from build123d import *

# Parameters (mm, degrees)
SKETCH_2_R        = 3.5
EXTRUDE_1_DEPTH   = 16
EXTRUDE_1_2_DEPTH = 16
EXTRUDE_1_3_DEPTH = 16
EXTRUDE_1_4_DEPTH = 16
SKETCH_3_W        = 288.1
SKETCH_3_H        = 15.5
EXTRUDE_2_DEPTH   = 15.5


with BuildPart() as part:
    # Sketch 2 → Extrude 1 (new body)
    with BuildSketch(Plane.XY):
        with Locations((-164, 0)):
            Circle(SKETCH_2_R)
    extrude(amount=EXTRUDE_1_DEPTH)



with BuildPart() as body_2:
    # Sketch 2 → Extrude 1 2 (new body)
    with BuildSketch(Plane.XY):
        with Locations((24.1, 0)):
            Circle(SKETCH_2_R)
    extrude(amount=EXTRUDE_1_2_DEPTH)


with BuildPart() as body_3:
    # Sketch 2 → Extrude 1 3 (new body)
    with BuildSketch(Plane.XY):
        with Locations((-204, 0)):
            Circle(SKETCH_2_R)
    extrude(amount=EXTRUDE_1_3_DEPTH)


with BuildPart() as body_4:
    # Sketch 2 → Extrude 1 4 (new body)
    with BuildSketch(Plane.XY):
        with Locations((64.1, 0)):
            Circle(SKETCH_2_R)
    extrude(amount=EXTRUDE_1_4_DEPTH)


with BuildPart() as part_1:
    add(part.part)

    add(body_2.part)  # Extrude 2 merges body 2

    add(body_3.part)  # Extrude 2 merges body 3

    add(body_4.part)  # Extrude 2 merges body 4
    # Sketch 3 → Extrude 2 (add)
    with BuildSketch(Plane(origin=(0, 0, 0), x_dir=(-1, 0, 0), z_dir=(0, 0, -1))):
        with Locations((69.95, 0)):
            Rectangle(SKETCH_3_W, SKETCH_3_H)
    extrude(amount=EXTRUDE_2_DEPTH)


solid = part_1.part
Work out the finished part from the listing and answer in its coordinate system (mm). A direction names the side the tool comes from. Give positions to 0.01 mm unless a question says otherwise; leave off trailing zeros. Order: outer loops, then holes, each group sorted by start corner. A loop starts at its lowest first (then second) coordinate and runs counter-clockwise, first axis right, second up. Notation, with made-up numbers: (39, -30) -> (93, -30) arc R23 ccw to (93, -5) -> close; hole circle Ø2 at (-9, 19). An arc over 180 degrees is marked (long way). Answer as a JSON object with one key per item and string values. Group by question number.
1. Section B-B on y = 0 is taken. Determine the outline of the cut face in (x, z), plus the area to 3 significant figures.
2. The mould has two halves that part along X. Classify faces 3 (the flat face through (24, 0, 16)), 4 (the cylindrical face through (67.333, -1.341, 7.888)), 5 (the flat face through (-214, 0, -8)), 6 (the flat face through (74.1, 0, -8)): released by +X, released by -X, zero draft, split by the parting line, or undercut.
3. Consider line 1 along X through (y, z) = (0.25, 1.5); line 2 along X through (y, z) = (3, 2.5); line 3 along Z through (x, y) = (-158, 0.5). Determine where each line is inside the solid, lowest interval first. Write a range as [from, to].
4. Section D-D on x = -125 is taken. Determine the outline of the cut face in (y, z), plus the area to 3 significant figures.
5. Section A-A on z = 11 is taken. Determine the outline of the cut face in (x, y), plus the area to 3 significant figures.
6. Section C-C on x = 64.1 is taken. Determine the outline of the cut face in (y, z), plus the area to 3 significant figures.
7. A flat-ended cylindrical pin translates along its axis: pin 1 Ø12 at (x, z) = (-146, 5) entering from +Y. Find the tip coordinate at first contact, or state that the pin passes through.
8. A tool of negligible diameter and unlimited length cuts with its end or side. For faces 1 (the cylindrical face through (-160.66, 1.05, 7.89)), 2 (the flat face through (64, 0, 16)), from which of +Z, -Z, +X, -X, +Y, -Y can it reach the whole face along a straight path? Write none if from no direction.
Result sheet:
{
 "1": {"outline": "(-214, -15.5) -> (74.1, -15.5) -> (74.1, 0) -> (67.6, 0) -> (67.6, 16) -> (60.6, 16) -> (60.6, 0) -> (27.6, 0) -> (27.6, 16) -> (20.6, 16) -> (20.6, 0) -> (-160.5, 0) -> (-160.5, 16) -> (-167.5, 16) -> (-167.5, 0) -> (-200.5, 0) -> (-200.5, 16) -> (-207.5, 16) -> (-207.5, 0) -> (-214, 0) -> close", "area": "4,910 mm^2"},
 "2": {"face 3": "zero draft", "face 4": "undercut", "face 5": "released by -X", "face 6": "released by +X"},
 "3": {"line 1": "x = [-207.49, -200.51], [-167.49, -160.51], [20.61, 27.59], [60.61, 67.59]", "line 2": "x = [-205.8, -202.2], [-165.8, -162.2], [22.3, 25.9], [62.3, 65.9]", "line 3": "z = [-15.5, 0]"},
 "4": {"outline": "(-7.75, -15.5) -> (7.75, -15.5) -> (7.75, 0) -> (-7.75, 0) -> close", "area": "240 mm^2"},
 "5": {"outline": "circle Ø7 at (-204, 0); circle Ø7 at (-164, 0); circle Ø7 at (24.1, 0); circle Ø7 at (64.1, 0)", "area": "154 mm^2"},
 "6": {"outline": "(-7.75, -15.5) -> (7.75, -15.5) -> (7.75, 0) -> (3.5, 0) -> (3.5, 16) -> (-3.5, 16) -> (-3.5, 0) -> (-7.75, 0) -> close", "area": "352 mm^2"},
 "7": {"pin 1": "stops at y = 7.75"},
 "8": {"face 1": "+Z", "face 2": "+Z, +X, -X, +Y, -Y"}
}
